```python
from build123d import *

# Parameters (mm, degrees)
SKETCH_1_R          = 1.25
EXTRUDE_1_DEPTH     = 4
EXTRUDE_2_DEPTH     = 4
SKETCH_3_R          = 1.25
EXTRUDE_3_DEPTH     = 2
SKETCH_4_R          = 2.6
CUT_EXTRUDE_1_DEPTH = 6
SKETCH_5_R          = 1.5
CUT_EXTRUDE_2_DEPTH = 37.100554012


with BuildPart() as part:
    # 草图1 → 凸台-拉伸1 (new body)
    with BuildSketch(Plane(origin=(0, 0, 0), x_dir=(1, 0, 0), z_dir=(0, 1, 0))):
        with BuildLine():
            Line((4.5, 9), (-4.5, 9))
            Line((-4.5, 9), (-6.675458936, 2.106714976))
            ThreePointArc((-6.675458936, 2.106714976), (-6.956816665, 0.776338774), (-6.9756521, -0.583333333))
            Line((-6.9756521, -0.583333333), (-4.484347779, -30.375))
            ThreePointArc((-4.484347779, -30.375), (0, -34.5), (4.484347779, -30.375))
            Line((4.484347779, -30.375), (6.9756521, -0.583333333))
            ThreePointArc((6.9756521, -0.583333333), (6.956816665, 0.776338774), (6.675458936, 2.106714976))
            Line((6.675458936, 2.106714976), (4.5, 9))
        make_face()
        with Locations(Location((0, -25, 0), (0, 0, 270))):
            Circle(SKETCH_1_R, mode=Mode.SUBTRACT)
        with Locations(Location((0, -20, 0), (0, 0, 270))):
            Circle(SKETCH_1_R, mode=Mode.SUBTRACT)
        with Locations(Location((0, -30, 0), (0, 0, 270))):
            Circle(SKETCH_1_R, mode=Mode.SUBTRACT)
    extrude(amount=EXTRUDE_1_DEPTH)

    # 草图2 → 凸台-拉伸2 (add)
    with BuildSketch(Plane(origin=(0, 4, 0), x_dir=(1, 0, 0), z_dir=(0, 1, 0))):
        with BuildLine():
            ThreePointArc((-6.675458936, 2.106714976), (-6.956816665, 0.776338774), (-6.9756521, -0.583333333))
            ThreePointArc((-6.9756521, -0.583333333), (0, -7), (6.9756521, -0.583333333))
            ThreePointArc((6.9756521, -0.583333333), (6.993910376, -0.291920622), (7, 0))
            ThreePointArc((7, 0), (6.918388994, 1.06578315), (6.675458936, 2.106714976))
            ThreePointArc((6.675458936, 2.106714976), (0, 7), (-6.675458936, 2.106714976))
        make_face()
        with BuildLine():
            Line((-4.5, 9), (-6.675458936, 2.106714976))
            ThreePointArc((-6.675458936, 2.106714976), (0, 7), (6.675458936, 2.106714976))
            Line((6.675458936, 2.106714976), (4.5, 9))
            Line((4.5, 9), (-4.5, 9))
        make_face()
    extrude(amount=EXTRUDE_2_DEPTH)

    # 草图3 → 凸台-拉伸3 (add)
    # profile 1 of 3: a face of its own
    with BuildSketch(Plane(origin=(0, 4, 0), x_dir=(1, 0, 0), z_dir=(0, 1, 0))):
        with BuildLine():
            Line((1, -16.980196905), (-1, -16.980196905))
            Line((-1, -16.980196905), (-1, -16.127016654))
            ThreePointArc((-1, -16.127016654), (-3.16227766, -17.550510257), (-4, -20))
            Line((-4, -20), (-4, -30))
            ThreePointArc((-4, -30), (0, -34), (4, -30))
            Line((4, -30), (4, -20))
            ThreePointArc((4, -20), (3.16227766, -17.550510257), (1, -16.127016654))
            Line((1, -16.127016654), (1, -16.980196905))
        make_face()
        with Locations(Location((0, -30, 0), (0, 0, 270))):
            Circle(SKETCH_3_R, mode=Mode.SUBTRACT)
        with Locations(Location((0, -25, 0), (0, 0, 270))):
            Circle(SKETCH_3_R, mode=Mode.SUBTRACT)
        with Locations(Location((0, -20, 0), (0, 0, 270))):
            Circle(SKETCH_3_R, mode=Mode.SUBTRACT)
    # profile 2 of 3: a face of its own
    with BuildSketch(Plane(origin=(0, 4, 0), x_dir=(1, 0, 0), z_dir=(0, 1, 0))):
        with BuildLine():
            Line((-1, -16.127016654), (-1, -16.980196905))
            Line((-1, -16.980196905), (1, -16.980196905))
            Line((1, -16.980196905), (1, -16.127016654))
            ThreePointArc((1, -16.127016654), (0, -16), (-1, -16.127016654))
        make_face()
    # profile 3 of 3: a face of its own
    with BuildSketch(Plane(origin=(0, 4, 0), x_dir=(1, 0, 0), z_dir=(0, 1, 0))):
        with BuildLine():
            Line((-1, -6.92820323), (-1, -16.127016654))
            ThreePointArc((-1, -16.127016654), (0, -16), (1, -16.127016654))
            Line((1, -16.127016654), (1, -6.92820323))
            ThreePointArc((1, -6.92820323), (0, -7), (-1, -6.92820323))
        make_face()
    extrude(amount=EXTRUDE_3_DEPTH)

    # 草图4 → 切除-拉伸1 (cut)
    with BuildSketch(Plane(origin=(0, 8, 0), x_dir=(1, 0, 0), z_dir=(0, 1, 0))):
        with Locations(Location((0, 0, 0), (0, 0, 270))):
            Circle(SKETCH_4_R)
    extrude(amount=-CUT_EXTRUDE_1_DEPTH, mode=Mode.SUBTRACT)

    # 草图5 → 切除-拉伸2 (cut, through all)
    with BuildSketch(Plane.XZ):
        with Locations(Location((0, 0, 0), (0, 0, 270))):
            Circle(SKETCH_5_R)
    extrude(amount=-CUT_EXTRUDE_2_DEPTH, mode=Mode.SUBTRACT)


solid = part.part
```
The listing builds one solid part. Answer for the finished solid, in the listing's coordinates (mm). A direction names the side the tool comes from. Give positions to 0.01 mm unless a question says otherwise; leave off trailing zeros. Order: outer loops, then holes, each group sorted by start corner. A loop starts at its lowest first (then second) coordinate and runs counter-clockwise, first axis right, second up. Notation, with made-up numbers: (21.25, -21.75) -> (44.25, -21.75) arc R33 cw to (44.25, 12.25) -> close; hole circle Ø1 at (-30.5, 31). An arc over 180 degrees is marked (long way). Answer as a JSON object with one key per item and string values. Group by question number.
Item 1: Consider L1, parallel to X at y = 4.35, z = 25; L2, parallel to X at y = 6.55, z = 0; L3, parallel to Z at x = 2, y = 6.5. Determine where each line is inside the solid, lowest interval first. Write a range as from..to.
Item 2: A tool of negligible diameter and unlimited length cuts with its end or side. For faces 1 (the cylindrical face through (-3.14, 4.99, 17.52)), 2 (the flat face through (1, 5, 12)), 3 (the flat face through (2, 4, 14)), 4 (the cylindrical face through (0, 5, 34)), 5 (the flat face through (4, 5, 25)), from which of +Z, -Z, +X, -X, +Y, -Y can it reach the whole face along a straight path? Write none if from no direction.
Item 3: Determine the mould class of faces 6 (the flat face through (-5.573, 3.944, -5.602)), 7 (the flat face through (-4, 5, 25)), 8 (the cylindrical face through (-0.479, 2.958, 21.155)), 9 (the cylindrical face through (-0.479, 2.958, 26.155)) for opening direction Z: pulls with the +Z half, pulls with the -Z half, needs draft (parallel to the pull), parting line crosses it, or undercut.
Item 4: The part is cut by section A-A on y = 0.5. Write down the section's boundary in (x, z) (3 decimals).
Item 5: The part is cut by section D-D on y = 3. Write down the section's boundary in (x, z) (3 decimals).
Item 6: The part is cut by section C-C on z = 9.5. Write down the section's boundary in (x, y).
Item 7: The part is cut by section B-B on x = 0. Write down the section's boundary in (y, z), and give its area (3 significant figures).
Item 8: Flat-ended cylindrical pins translate along their axes: pin 1 (7 mm diameter, centred on x = 0, z = 0, fed in from +Y); pin 2 (2 mm diameter, centred on x = 0, z = 20, fed in from -Y); pin 3 (2.5 mm diameter, centred on x = -1, z = 18.5, fed in from +Y); pin 4 (1.5 mm diameter, centred on y = 3, z = 24.5, fed in from +X). Find the tip coordinate at first contact, or state that the pin passes through.
Result set:
{
 "1": {"L1": "-4..-1.25, 1.25..4", "L2": "-7..-2.6, 2.6..7", "L3": "-9..-1.66, 1.66..6.71"},
 "2": {"face 1": "-X, +Y", "face 2": "+X, +Y", "face 3": "+Y", "face 4": "+Z, +Y", "face 5": "+Z, +X, +Y"},
 "3": {"face 6": "pulls with the -Z half", "face 7": "needs draft", "face 8": "undercut", "face 9": "undercut"},
 "4": {"outline": "(-6.976, 0.583) arc R7 ccw to (-6.675, -2.107) -> (-4.5, -9) -> (4.5, -9) -> (6.675, -2.107) arc R7 ccw to (6.976, 0.583) -> (4.484, 30.375) arc R4.5 ccw to (-4.484, 30.375) -> close; hole circle Ø3 at (0, 0); hole circle Ø2.5 at (0, 20); hole circle Ø2.5 at (0, 25); hole circle Ø2.5 at (0, 30)"},
 "5": {"outline": "(-6.976, 0.583) arc R7 ccw to (-6.675, -2.107) -> (-4.5, -9) -> (4.5, -9) -> (6.675, -2.107) arc R7 ccw to (6.976, 0.583) -> (4.484, 30.375) arc R4.5 ccw to (-4.484, 30.375) -> close; hole circle Ø5.2 at (0, 0); hole circle Ø2.5 at (0, 20); hole circle Ø2.5 at (0, 25); hole circle Ø2.5 at (0, 30)"},
 "6": {"outline": "(-6.23, 0) -> (6.23, 0) -> (6.23, 4) -> (1, 4) -> (1, 6) -> (-1, 6) -> (-1, 4) -> (-6.23, 4) -> close"},
 "7": {"outline": "(0, -9) -> (8, -9) -> (8, -2.6) -> (2, -2.6) -> (2, -1.5) -> (0, -1.5) -> close; (0, 1.5) -> (2, 1.5) -> (2, 2.6) -> (8, 2.6) -> (8, 7) -> (6, 7) -> (6, 18.75) -> (0, 18.75) -> close; (0, 21.25) -> (6, 21.25) -> (6, 23.75) -> (0, 23.75) -> close; (0, 26.25) -> (6, 26.25) -> (6, 28.75) -> (0, 28.75) -> close; (0, 31.25) -> (6, 31.25) -> (6, 34) -> (4, 34) -> (4, 34.5) -> (0, 34.5) -> close", "area": "210 mm²"},
 "8": {"pin 1": "y = 8", "pin 2": "through", "pin 3": "y = 6", "pin 4": "x = 5.04"}
}
